The drawing under review shows one solid part. Ordinate dimensions are in mm from its lowest x, y, z. Round coordinates to 2 decimals unless told otherwise and drop trailing zeros. Order: outer loops, then holes, each group sorted by start corner. A loop starts at its lowest first (then second) coordinate and runs counter-clockwise, first axis right, second up.
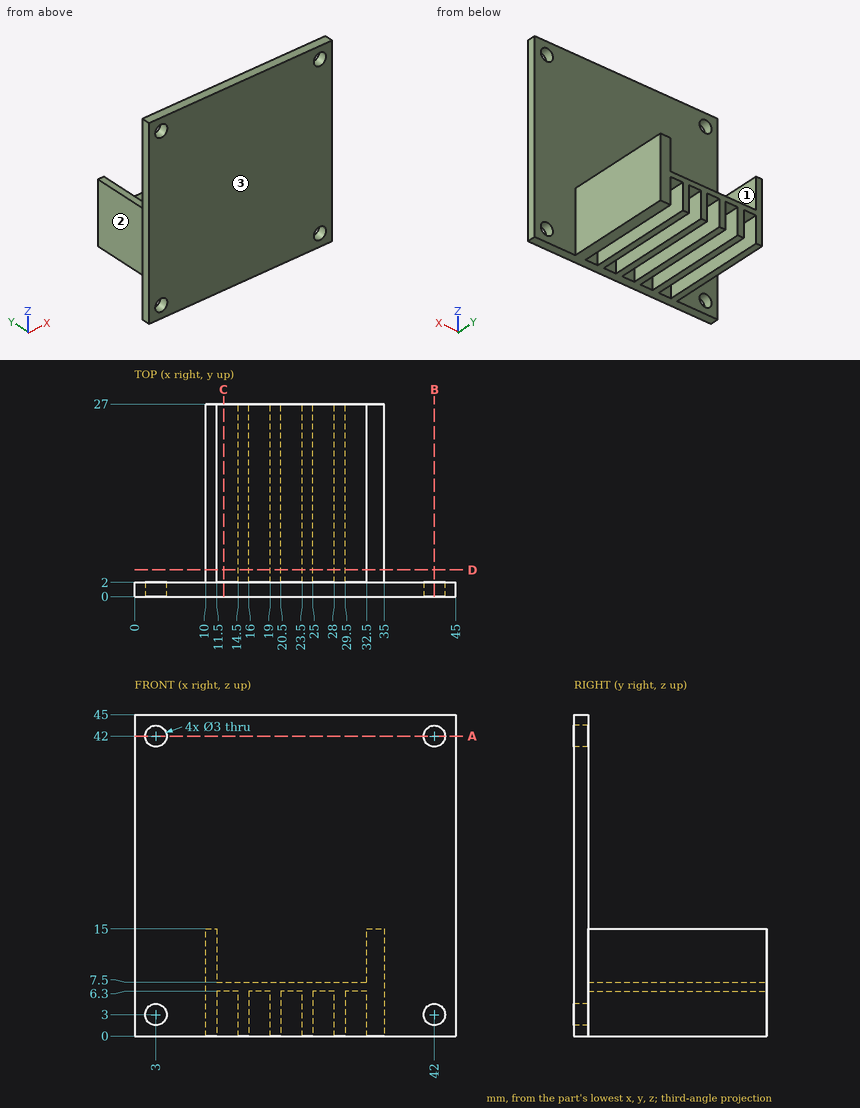
Q1. Wall thickness on line 1 (Z direction, x = 42, y = 0.85); line 2 (X direction, y = 6.25, z = 6): over which ranges is each line inside the solid? List them lowest first.
Q2. Mouldability with a two-part tool opening along X and no side actions: class the marked faces 1, 2 and 3 as +X half, -X half, draft (parallel to the pull), parting line (faces both ways), or undercut.
Q3. Take a section at B-B, the plane x = 42. State the section outline as (y, z) points, plus the area to 3 significant figures.
Q4. Take a section at C-C, the plane x = 12.5. State the section outline as (y, z) points, plus the area to 3 significant figures.
Q5. Take a section at D-D, the plane y = 3.75. State the section outline as (x, z) points, plus the area to 3 significant figures.
Q6. Clearance check with flat-ended pins moving along their axes: pin 1 (6 mm diameter, centred on y = 22, z = 6, fed in from -X); pin 2 (3 mm diameter, centred on y = 20, z = 4.5, fed in from +X); pin 3 (1.5 mm diameter, centred on x = 26.5, y = 14, fed in from -Z). State where each tip first meets the part, or that it passes through.
Q7. Take a section at A-A, the plane z = 42. State the section outline as (x, y) points, plus the area to 3 significant figures.
Working result:
1. line 1: z = 0 to 1.5, 4.5 to 40.5, 43.5 to 45
1. line 2: x = 10 to 11.5, 14.5 to 16, 19 to 20.5, 23.5 to 25, 28 to 29.5, 32.5 to 35
2. face 1: undercut
2. face 2: -X half
2. face 3: draft
3. outline: (0, 0) - (2, 0) - (2, 1.5) - (0, 1.5) - close; (0, 4.5) - (2, 4.5) - (2, 40.5) - (0, 40.5) - close; (0, 43.5) - (2, 43.5) - (2, 45) - (0, 45) - close
3. area: 78.0 mm2
4. outline: (0, 0) - (2, 0) - (2, 6.3) - (27, 6.3) - (27, 7.5) - (2, 7.5) - (2, 45) - (0, 45) - close
4. area: 120 mm2
5. outline: (10, 0) - (11.5, 0) - (11.5, 6.3) - (14.5, 6.3) - (14.5, 0) - (16, 0) - (16, 6.3) - (19, 6.3) - (19, 0) - (20.5, 0) - (20.5, 6.3) - (23.5, 6.3) - (23.5, 0) - (25, 0) - (25, 6.3) - (28, 6.3) - (28, 0) - (29.5, 0) - (29.5, 6.3) - (32.5, 6.3) - (32.5, 0) - (35, 0) - (35, 15) - (32.5, 15) - (32.5, 7.5) - (11.5, 7.5) - (11.5, 15) - (10, 15) - close
5. area: 123 mm2
6. pin 1: stops at x = 10
6. pin 2: stops at x = 35
6. pin 3: stops at z = 6.3
7. outline: (0, 0) - (1.5, 0) - (1.5, 2) - (0, 2) - close; (4.5, 0) - (40.5, 0) - (40.5, 2) - (4.5, 2) - close; (43.5, 0) - (45, 0) - (45, 2) - (43.5, 2) - close
7. area: 78.0 mm2
